Read the model definition and answer for the solid it produces. Units are mm, in the model's axes. A direction names the side the tool comes from. Coordinates: 2 decimals unless noted, no trailing zeros. Write each loop counter-clockwise with the first axis right and the second up, starting at its lowest first coordinate (ties: lowest second). Pieces come first, ordered by that corner, then holes. Notation, with made-up numbers: (75, 27.25) -> (107, 27.25) arc R21 ccw to (107, 36.25) -> close; hole circle Ø8 at (5, -2). An arc over 180 degrees is marked (long way). Answer as a JSON object with one key per item and string values. Group by question number.
(1) Find section A-A (z = 15). Give the vertices of the cut face in (x, y) (3 decimals).
(2) Find section B-B (x = 0). Give the vertices of the cut face in (y, z) (3 decimals), then the cut area to 3 significant figures.
(3) Find section D-D (z = 2.75). Give the vertices of the cut face in (x, y) (3 decimals), then the cut area to 3 significant figures.
(4) Which of the six approach directions +Z, -Z, +X, -X, +Y, -Y give full straight-line access (tool end or side, diameter ignored) to faces 1 (the face through (1.537, 6, 19)), 2 (the face through (2, 2.3, 0))?
(5) For a pull along Y with two mould halves and no side action, classify faces 3 (the face through (-2.06, -9.3, 12.52)), 4 (the face through (-2.79, 0.12, 9.7)), 5 (the face through (-5, 0, 25.4)) as +Y half, -Y half, draft (parallel to the pull), parting line (faces both ways), or undercut.
(6) Straight lines are drawn through the part: L1, parallel to Y at x = 0, z = 9.25 (3 decimals); L2, parallel to Z at x = -0.75, y = 2.75; L3, parallel to X at y = 1.5, z = 17.5. For each, find the intervals that lie inside material, in ascending order.
(7) Find section C-C (y = 4). Give the vertices of the cut face in (x, z).
(8) Flat-ended cylindrical pins translate along their axes: P1, Ø2, axis at x = 4.5, z = 6, coming from the +Y side; P2, Ø5.5, axis at y = -5.5, z = 20.5, coming from the +X side; P3, Ø3.5, axis at y = 7, z = 22, coming from the +X side. Find the tip coordinate at first contact, or state that the pin passes through.
from build123d import *

# Parameters (mm, degrees)
F0_R     = 9.525
F0_R_2   = 2.794
F1_DEPTH = 25.4
F2_W     = 3.0734
F2_H     = 25.4
F3_DEPTH = 12.7
F4_DEPTH = 25.4


with BuildPart() as f1:
    # F0 (on Top) → F1 (new body)
    with BuildSketch(Plane.XY):
        Circle(F0_R)
        Circle(F0_R_2, mode=Mode.SUBTRACT)
        Circle(F0_R_2)
    extrude(amount=F1_DEPTH)

    # F2 (on Front) → F3 (cut, symmetric)
    with BuildSketch(Plane.XZ):
        with Locations((0, 25.4)):
            Rectangle(F2_W, F2_H)
    extrude(amount=F3_DEPTH, both=True, mode=Mode.SUBTRACT)

    # F0 (on Top) → F4 (cut, through all)
    with BuildSketch(Plane.XY):
        Circle(F0_R_2)
    extrude(amount=F4_DEPTH, mode=Mode.SUBTRACT)


solid = f1.part
Results below:
{
 "1": {"outline": "(-1.537, -9.4) -> (-1.537, -2.333) arc R2.794 cw to (-1.537, 2.333) -> (-1.537, 9.4) arc R9.525 ccw to start; (1.537, -9.4) arc R9.525 ccw to (1.537, 9.4) -> (1.537, 2.333) arc R2.794 cw to (1.537, -2.333) -> close"},
 "2": {"outline": "(-9.525, 0) -> (-2.794, 0) -> (-2.794, 12.7) -> (-9.525, 12.7) -> close; (2.794, 0) -> (9.525, 0) -> (9.525, 12.7) -> (2.794, 12.7) -> close", "area": "171 mm2"},
 "3": {"outline": "circle Ø19.05 at (0, 0); hole circle Ø5.588 at (0, 0)", "area": "260 mm2"},
 "4": {"face 1": "+Z, +Y, -Y", "face 2": "-Z, +X, -X, +Y, -Y"},
 "5": {"face 3": "parting line", "face 4": "undercut", "face 5": "draft"},
 "6": {"L1": "y = -9.525 to -2.794, 2.794 to 9.525", "L2": "z = 0 to 12.7", "L3": "x = -9.41 to -2.36, 2.36 to 9.41"},
 "7": {"outline": "(-8.64, 0) -> (8.64, 0) -> (8.64, 25.4) -> (1.54, 25.4) -> (1.54, 12.7) -> (-1.54, 12.7) -> (-1.54, 25.4) -> (-8.64, 25.4) -> close"},
 "8": {"P1": "stops at y = 8.86", "P2": "stops at x = 9.12", "P3": "stops at x = 7.95"}
}
